Autodesk Inventor part; units mm, degrees
ref_plane "YZ Plane" through (0, 0, 0) normal (1, 0, 0) x (0, 1, 0)
ref_plane "XZ Plane" through (0, 0, 0) normal (0, 1, 0) x (-1, 0, 0)
ref_plane "XY Plane" through (0, 0, 0) normal (0, 0, 1) x (1, 0, 0)
sketch "Sketch4" plane through (0, 0, 0) normal (0, 1, 0) x (-1, 0, 0)
  circle A0 centre (0, 0) radius 32.5
  line L0 (85.3525, 23.3053) -> (40.3525, 23.3053)
  line L1 (40.3525, 23.3053) -> (40.3525, -21.6947)
  line L2 (40.3525, -21.6947) -> (85.3525, -21.6947)
  line L3 (85.3525, -21.6947) -> (85.3525, 23.3053)
  line L4 (22.4932, 85.5701) -> (-0.0068, 46.5989)
  line L5 (-0.0068, 46.5989) -> (38.9644, 24.0989)
  line L6 (38.9644, 24.0989) -> (61.4644, 63.0701)
  line L7 (61.4644, 63.0701) -> (22.4932, 85.5701)
  line L8 (-62.8593, 62.2648) -> (-40.3593, 23.2936)
  line L9 (-40.3593, 23.2936) -> (-1.3881, 45.7936)
  line L10 (-1.3881, 45.7936) -> (-23.8881, 84.7648)
  line L11 (-23.8881, 84.7648) -> (-62.8593, 62.2648)
  line L12 (-85.3525, -23.3053) -> (-40.3525, -23.3053)
  line L13 (-40.3525, -23.3053) -> (-40.3525, 21.6947)
  line L14 (-40.3525, 21.6947) -> (-85.3525, 21.6947)
  line L15 (-85.3525, 21.6947) -> (-85.3525, -23.3053)
  line L16 (-22.4932, -85.5701) -> (0.0068, -46.5989)
  line L17 (0.0068, -46.5989) -> (-38.9644, -24.0989)
  line L18 (-38.9644, -24.0989) -> (-61.4644, -63.0701)
  line L19 (-61.4644, -63.0701) -> (-22.4932, -85.5701)
  line L20 (62.8593, -62.2648) -> (40.3593, -23.2936)
  line L21 (40.3593, -23.2936) -> (1.3881, -45.7936)
  line L22 (1.3881, -45.7936) -> (23.8881, -84.7648)
  line L23 (23.8881, -84.7648) -> (62.8593, -62.2648)
  circle A1 centre (0, 0) radius 91
  line L24 (0, -32.5) -> (0, -91)
  dimension "d5" = 65
  dimension "d12" = 182
  dimension "d6" = 45
  dimension "d7" = 45
  dimension "d10" = 360
extrude "Extrusion2" add sketch "Sketch4" against normal blind 1.2 contours A0 | A1 | L17 L16 L24 | L24 L16 L19 L18 L17 | L3 L2 L1 L0 | L7 L6 L5 L4 | L11 L10 L9 L8 | L15 L14 L13 L12 | L23 L22 L21 L20
sketch "Sketch6" plane through (0, 0, 0) normal (0, 1, 0) x (1, 0, 0)
  circle A0 centre (0, 0) radius 42.5
  circle A1 centre (0, 0) radius 91
  line L0 (-0.7102, 83.7173) -> (0.2898, 83.7173)
  line L1 (0.2898, 83.7173) -> (0.2898, 43.1226)
  line L2 (0.2898, 43.1226) -> (-0.7102, 43.1226)
  line L3 (-0.7102, 43.1226) -> (-0.7102, 83.7173)
  dimension "d15" = 85
  dimension "d16" = 1
extrude "Extrusion3" add sketch "Sketch6" along normal blind 10 contours L0 L1 L2 L3
pattern_circular "Circular Pattern1" count 6 over 360 about axis through (0, -10, 0) along (0, 1, 0) of "Extrusion3"
sketch "Sketch7" plane through (0, 0, 0) normal (0, 1, 0) x (1, 0, 0)
  circle A0 centre (0, 0) radius 32.5
  dimension "d24" = 65
extrude "Extrusion4" add sketch "Sketch7" along normal blind 10
sketch "Sketch12" plane through (0, 10, 0) normal (0, 1, 0) x (1, 0, 0)
  point P0 (0, 0)
  point P1 (0, 0)
hole "Hole3" at (0, 10, 0) direction (0, -1, 0) diameter 63 depth 10
sketch "Sketch13" plane through (0, 0, 0) normal (0, 1, 0) x (1, 0, 0)
  point P0 (0, 0)
  point P1 (0, 0)
hole "Hole4" at (0, 0, 0) direction (0, -1, 0) diameter 5 depth 2
properties part number "Plate"
Model file for the job. Use its own axes, mm. A direction names the side the tool comes from. Round coordinates to 2 decimals unless told otherwise and drop trailing zeros. Order: outer loops, then holes, each group sorted by start corner. A loop starts at its lowest first (then second) coordinate and runs counter-clockwise, first axis right, second up. Notation, with made-up numbers: M 44,60 L 93,60 A23 cw 93,99 Z; hole C 80.25,-29 d3. An arc over 180 degrees is marked long. Write each question's results on one line, items separated by ' | '. Start each with the question number.
(1) Probe probe 1 along Z at (x, y) = (0, 8); probe 2 along Z at (x, y) = (0, -0.65); probe 3 along X at (y, z) = (7.75, 0). List the from-to ranges inside material, lowest first. Write a range as from..to.
(2) Which spindle directions (+Z, -Z, +X, -X, +Y, -Y) get a long thin tool onto all of the face, cutting with end or side? Do faces 5 (the face through (55.03, 4.93, 30.95)), 6 (the face through (-55.03, 4.93, -30.95)), 7 (the face through (-0.71, 5, -63)), 8 (the face through (0.71, 5, 63)). Say none if no direction does.
(3) Saw through at D-D, the plane z = -59.5. Give the cut face in (x, y).
(4) Saw through at B-B, the plane z = -10. Give the cut face in (x, y), then the cut area to 3 significant figures.
(5) Saw through at C-C, the plane x = 68.5. Give the cut face in (y, z).
(6) Drop flat-ended pins along their axis: pin 1 (6 mm diameter, centred on x = -56, y = 0, fed in from -Z); pin 2 (3 mm diameter, centred on x = 50.5, z = -62, fed in from +Y); pin 3 (1 mm diameter, centred on y = 3.5, z = 6, fed in from -X); pin 4 (4.5 mm diameter, centred on x = 0, z = 0, fed in from -Y). Give the stop position or say it passes through.
(7) Two-plate mould, pull along X, no slides. Class faces 1 (the face through (72.214, -0.592, -55.372)), 2 (the face through (0, 0, 7)), 3 (the face through (54.32, 4.93, -32.18)), 4 (the face through (-19, -1.2, 1)): pulls with the +X half, pulls with the -X half, needs draft (parallel to the pull), parting line crosses it, or undercut.
(8) Saw through at A-A, the plane y = 7.5. Give the cut face in (x, z).
Established:
1) probe 1: z = -83.72..-43.12, -32.5..-31.5, 31.5..32.5, 43.12..83.72 | probe 2: z = -91..-2.5, 2.5..91 | probe 3: x = -32.5..-31.5, 31.5..32.5
2) face 5: +X, +Y | face 6: -X, +Y | face 7: -Z, -X, +Y | face 8: +Z, +X, +Y
3) outline: M -68.85,-1.2 L 68.85,-1.2 L 68.85,0 L 0.29,0 L 0.29,10 L -0.71,10 L -0.71,0 L -68.85,0 Z
4) outline: M -90.45,-1.2 L 90.45,-1.2 L 90.45,0 L 30.92,0 L 30.92,10 L 29.87,10 L 29.87,0 L -29.87,0 L -29.87,10 L -30.92,10 L -30.92,0 L -90.45,0 Z | area: 238 mm^2
5) outline: M -1.2,-59.91 L 0,-59.91 L 0,-40.37 L 10,-40.37 L 10,-39.21 L 0,-39.21 L 0,38.73 L 10,38.73 L 10,39.88 L 0,39.88 L 0,59.91 L -1.2,59.91 Z
6) pin 1: stops at z = -73.97 | pin 2: stops at y = 0 | pin 3: stops at x = -32.03 | pin 4: passes through
7) face 1: parting line crosses it | face 2: undercut | face 3: undercut | face 4: needs draft
8) outline: M -72.86,-41.24 L -72.36,-42.11 L -37.2,-21.81 L -37.7,-20.95 Z; M -72.65,41.61 L -37.49,21.31 L -36.99,22.18 L -72.15,42.47 Z; C 0,0 d65; M -0.71,-83.72 L 0.29,-83.72 L 0.29,-43.12 L -0.71,-43.12 Z; M -0.29,43.12 L 0.71,43.12 L 0.71,83.72 L -0.29,83.72 Z; M 36.99,-22.18 L 72.15,-42.47 L 72.65,-41.61 L 37.49,-21.31 Z; M 37.2,21.81 L 37.7,20.95 L 72.86,41.24 L 72.36,42.11 Z; hole C 0,0 d63
